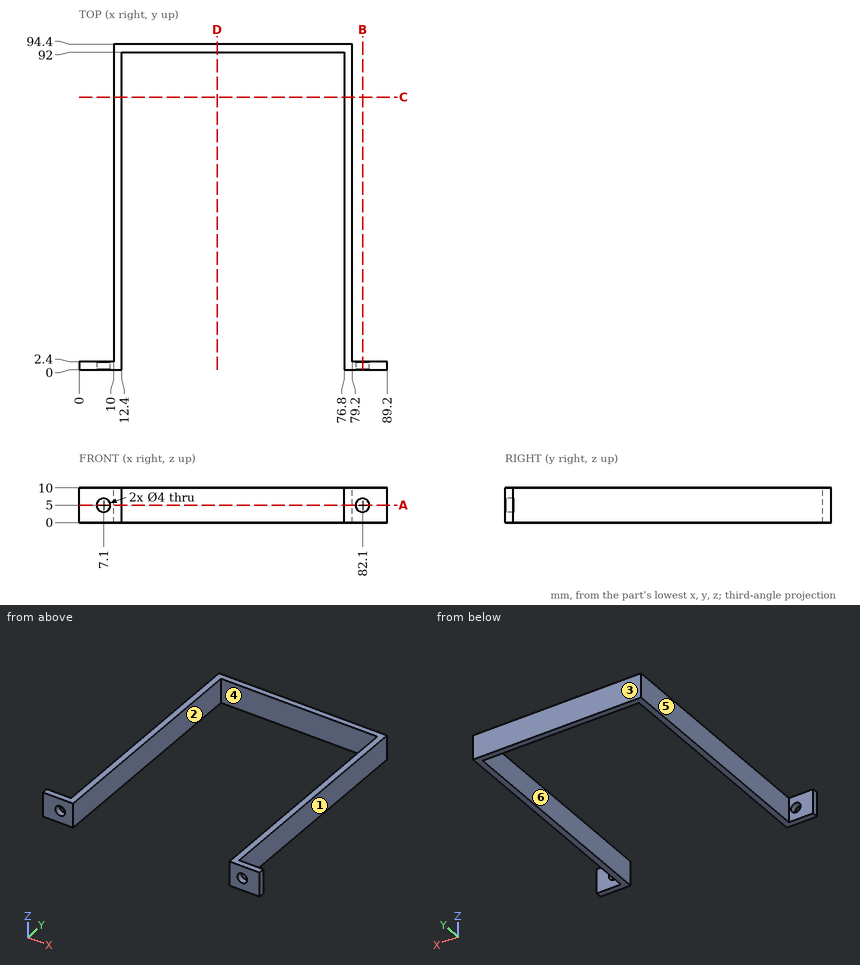
Drawing for the job (mm, zero at the part's lowest x, y, z). A direction names the side the tool comes from. Round coordinates to 2 decimals unless told otherwise and drop trailing zeros. Write each loop counter-clockwise with the first axis right and the second up, starting at its lowest first coordinate (ties: lowest second). Pieces come first, ordered by that corner, then holes.
Item 1: Tool access for the marked faces 1 and 2: list every direction of +Z, -Z, +X, -X, +Y, -Y with a clear straight run to the whole face (end or side of a thin tool).
Filled in:
face 1: +Z, -Z, +X, +Y
face 2: +Z, -Z, -Y
Item 2: Drill centre lines: L1, parallel to Z at x = 7.1, y = 0.85; L2, parallel to X at y = 66, z = 4.25; L3, parallel to Y at x = 73.5, z = 9.5. Where is each one in solid material? Low to high.
Filled in:
L1: z = 0 to 3, 7 to 10
L2: x = 10 to 12.4, 76.8 to 79.2
L3: y = 92 to 94.4
Item 3: Drop flat-ended pins along their axis: pin 1 Ø6 at (y, z) = (57, 6) entering from +X; pin 2 Ø3 at (x, z) = (82.1, 5) entering from +Y; pin 3 Ø5 at (x, z) = (3, 7) entering from +Y; pin 4 Ø5 at (y, z) = (29, 3.5) entering from -X. Give the stop position or say it passes through.
Filled in:
pin 1: stops at x = 79.2
pin 2: passes through
pin 3: stops at y = 2.4
pin 4: stops at x = 10
Item 4: Band-saw the part on A-A on z = 5. Write the cut outline in (x, y), then the cut area to 3 significant figures.
Filled in:
outline: (0, 0) - (5.1, 0) - (5.1, 2.4) - (0, 2.4) - close; (9.1, 0) - (12.4, 0) - (12.4, 92) - (76.8, 92) - (76.8, 0) - (80.1, 0) - (80.1, 2.4) - (79.2, 2.4) - (79.2, 94.4) - (10, 94.4) - (10, 2.4) - (9.1, 2.4) - close; (84.1, 0) - (89.2, 0) - (89.2, 2.4) - (84.1, 2.4) - close
area: 636 mm2
Item 5: Band-saw the part on B-B on x = 82.1. Write the cut outline in (y, z), then the cut area to 3 significant figures.
Filled in:
outline: (0, 0) - (2.4, 0) - (2.4, 3) - (0, 3) - close; (0, 7) - (2.4, 7) - (2.4, 10) - (0, 10) - close
area: 14.4 mm2
Item 6: Band-saw the part on C-C on y = 79. Write the cut outline in (x, z).
Filled in:
outline: (10, 0) - (12.4, 0) - (12.4, 10) - (10, 10) - close; (76.8, 0) - (79.2, 0) - (79.2, 10) - (76.8, 10) - close
Item 7: Mould opens along X. For the marked faces 3, 4, 5 and 6 say: released by +X, released by -X, zero draft, split by the parting line, or undercut.
Filled in:
face 3: zero draft
face 4: undercut
face 5: released by -X
face 6: undercut
Item 8: Band-saw the part on D-D on x = 40. Write the cut outline in (y, z), then the cut area to 3 significant figures.
Filled in:
outline: (92, 0) - (94.4, 0) - (94.4, 10) - (92, 10) - close
area: 24.0 mm2
